```python
from build123d import *

# Parameters (mm, degrees)
SKETCH1_W           = 26.67
SKETCH1_H           = 6.858
BOSS_EXTRUDE1_DEPTH = 5.588
CUT_EXTRUDE1_REACH  = 184.177
SKETCH9_W           = 6.096
SKETCH9_H           = 12.7
CUT_EXTRUDE2_REACH  = 184.177
SKETCH12_R          = 3.175
CUT_EXTRUDE3_REACH  = 184.177
SKETCH13_R          = 4.445


with BuildPart() as part:
    # Sketch1 → Boss-Extrude1 (new body)
    with BuildSketch(Plane(origin=(0, 0, 0), x_dir=(1, 0, 0), z_dir=(0, 1, 0))):
        Polygon((-110.690062624, 12.380140685), (-116.278062624, 12.380140685), (-116.278062624, 0.950140685), (-110.690062624, 0.950140685), (-110.690062624, -46.674859251), (-97.228062624, -46.674859251), (-97.228062624, -52.262859251), (-85.798062624, -52.262859251), (-85.798062624, -46.674859251), (-59.128062624, -46.674859251), (-59.128062624, -52.262859251), (-15.948062624, -52.262859251), (-15.948062624, -46.674859251), (10.721937376, -46.674859251), (10.721937376, -52.262859251), (72.951937376, -52.262859251), (72.951937376, -46.674859251), (99.621937376, -46.674859251), (99.621937376, -52.262859251), (130.101937376, -52.262859251), (130.101937376, -46.67485938), (143.563937376, -46.67485938), (143.563937376, 0.950140682), (149.151937376, 0.950140682), (149.151937376, 12.38014062), (143.563937376, 12.38014062), (143.563937376, 60.00514062), (130.101937376, 60.00514062), (130.101937376, 66.86314062), (143.563937376, 66.86314062), (143.563937376, 104.45514062), (-105.610062624, 104.45514062), (-105.610062624, 66.86314062), (-97.228062624, 66.86314062), (-97.228062624, 60.00514062), (-110.690062624, 60.00514062), align=None)
        with Locations((-72.463062624, 63.43414062)):
            Rectangle(SKETCH1_W, SKETCH1_H, mode=Mode.SUBTRACT)
        with Locations((-2.613062624, 63.43414062)):
            Rectangle(SKETCH1_W, SKETCH1_H, mode=Mode.SUBTRACT)
        with Locations((86.286937376, 63.43414062)):
            Rectangle(SKETCH1_W, SKETCH1_H, mode=Mode.SUBTRACT)
    extrude(amount=BOSS_EXTRUDE1_DEPTH)

    # Sketch9 → Cut-Extrude1 (cut, up to next)
    with BuildSketch(Plane(origin=(0, 5.588, 0), x_dir=(1, 0, 0), z_dir=(0, 1, 0)), mode=Mode.PRIVATE) as cut_extrude1_sk1:
        with Locations((-20.012062624, -23.687859251)):
            Rectangle(SKETCH9_W, SKETCH9_H)
    cut_extrude1_tool1 = extrude(cut_extrude1_sk1.sketch, amount=-CUT_EXTRUDE1_REACH, mode=Mode.PRIVATE) & part.part
    # Sketch9 → Cut-Extrude1 (cut, up to next)
    with BuildSketch(Plane(origin=(0, 5.588, 0), x_dir=(1, 0, 0), z_dir=(0, 1, 0)), mode=Mode.PRIVATE) as cut_extrude1_sk2:
        with Locations((-20.012062624, 42.860140749)):
            Rectangle(SKETCH9_W, SKETCH9_H)
    cut_extrude1_tool2 = extrude(cut_extrude1_sk2.sketch, amount=-CUT_EXTRUDE1_REACH, mode=Mode.PRIVATE) & part.part
    # Sketch9 → Cut-Extrude1 (cut, up to next)
    with BuildSketch(Plane(origin=(0, 5.588, 0), x_dir=(1, 0, 0), z_dir=(0, 1, 0)), mode=Mode.PRIVATE) as cut_extrude1_sk3:
        with Locations((133.657937376, -23.687859251)):
            Rectangle(SKETCH9_W, SKETCH9_H)
    cut_extrude1_tool3 = extrude(cut_extrude1_sk3.sketch, amount=-CUT_EXTRUDE1_REACH, mode=Mode.PRIVATE) & part.part
    # Sketch9 → Cut-Extrude1 (cut, up to next)
    with BuildSketch(Plane(origin=(0, 5.588, 0), x_dir=(1, 0, 0), z_dir=(0, 1, 0)), mode=Mode.PRIVATE) as cut_extrude1_sk4:
        with Locations((133.657937376, 42.860140749)):
            Rectangle(SKETCH9_W, SKETCH9_H)
    cut_extrude1_tool4 = extrude(cut_extrude1_sk4.sketch, amount=-CUT_EXTRUDE1_REACH, mode=Mode.PRIVATE) & part.part
    add(cut_extrude1_tool1.solids().sort_by_distance((-20.012063, 5.588, 23.687859))[0], mode=Mode.SUBTRACT)
    add(cut_extrude1_tool2.solids().sort_by_distance((-20.012063, 5.588, -42.860141))[0], mode=Mode.SUBTRACT)
    add(cut_extrude1_tool3.solids().sort_by_distance((133.657937, 5.588, 23.687859))[0], mode=Mode.SUBTRACT)
    add(cut_extrude1_tool4.solids().sort_by_distance((133.657937, 5.588, -42.860141))[0], mode=Mode.SUBTRACT)

    # Sketch12 → Cut-Extrude2 (cut, up to next)
    with BuildSketch(Plane(origin=(0, 5.588, 0), x_dir=(1, 0, 0), z_dir=(0, 1, 0)), mode=Mode.PRIVATE) as cut_extrude2_sk1:
        with Locations(Location((-101.165062624, 28.25514062, 0), (0, 0, 270))):
            Circle(SKETCH12_R)
    cut_extrude2_tool1 = extrude(cut_extrude2_sk1.sketch, amount=-CUT_EXTRUDE2_REACH, mode=Mode.PRIVATE) & part.part
    add(cut_extrude2_tool1.solids().sort_by_distance((-101.165063, 5.588, -28.255141))[0], mode=Mode.SUBTRACT)

    # Sketch13 → Cut-Extrude3 (cut, up to next)
    with BuildSketch(Plane.XZ, mode=Mode.PRIVATE) as cut_extrude3_sk1:
        with Locations(Location((77.273937376, 20.297859251, 0), (0, 0, 270))):
            Circle(SKETCH13_R)
    cut_extrude3_tool1 = extrude(cut_extrude3_sk1.sketch, amount=-CUT_EXTRUDE3_REACH, mode=Mode.PRIVATE) & part.part
    # Sketch13 → Cut-Extrude3 (cut, up to next)
    with BuildSketch(Plane.XZ, mode=Mode.PRIVATE) as cut_extrude3_sk2:
        with Locations(Location((55.099783131, -40.95514062, 0), (0, 0, 270))):
            Circle(SKETCH13_R)
    cut_extrude3_tool2 = extrude(cut_extrude3_sk2.sketch, amount=-CUT_EXTRUDE3_REACH, mode=Mode.PRIVATE) & part.part
    # Sketch13 → Cut-Extrude3 (cut, up to next)
    with BuildSketch(Plane.XZ, mode=Mode.PRIVATE) as cut_extrude3_sk3:
        with Locations(Location((94.474354319, -40.95514062, 0), (0, 0, 270))):
            Circle(SKETCH13_R)
    cut_extrude3_tool3 = extrude(cut_extrude3_sk3.sketch, amount=-CUT_EXTRUDE3_REACH, mode=Mode.PRIVATE) & part.part
    # Sketch13 → Cut-Extrude3 (cut, up to next)
    with BuildSketch(Plane.XZ, mode=Mode.PRIVATE) as cut_extrude3_sk4:
        with Locations(Location((75.424354319, -15.55514062, 0), (0, 0, 270))):
            Circle(SKETCH13_R)
    cut_extrude3_tool4 = extrude(cut_extrude3_sk4.sketch, amount=-CUT_EXTRUDE3_REACH, mode=Mode.PRIVATE) & part.part
    # Sketch13 → Cut-Extrude3 (cut, up to next)
    with BuildSketch(Plane.XZ, mode=Mode.PRIVATE) as cut_extrude3_sk5:
        with Locations(Location((29.478937376, -48.367787821, 0), (0, 0, 270))):
            Circle(SKETCH13_R)
    cut_extrude3_tool5 = extrude(cut_extrude3_sk5.sketch, amount=-CUT_EXTRUDE3_REACH, mode=Mode.PRIVATE) & part.part
    add(cut_extrude3_tool1.solids().sort_by_distance((77.273937, 0, 20.297859))[0], mode=Mode.SUBTRACT)
    add(cut_extrude3_tool2.solids().sort_by_distance((55.099783, 0, -40.955141))[0], mode=Mode.SUBTRACT)
    add(cut_extrude3_tool3.solids().sort_by_distance((94.474354, 0, -40.955141))[0], mode=Mode.SUBTRACT)
    add(cut_extrude3_tool4.solids().sort_by_distance((75.424354, 0, -15.555141))[0], mode=Mode.SUBTRACT)
    add(cut_extrude3_tool5.solids().sort_by_distance((29.478937, 0, -48.367788))[0], mode=Mode.SUBTRACT)


solid = part.part
```
Verification items for the finished model (mm, model axes). A direction names the side the tool comes from. Coordinates: 2 decimals unless noted, no trailing zeros. Order: outer loops, then holes, each group sorted by start corner. A loop starts at its lowest first (then second) coordinate and runs counter-clockwise, first axis right, second up. Notation, with made-up numbers: (38, 68) -> (71, 68) arc R29 ccw to (71, 93) -> close; hole circle Ø1 at (-32, 29.25). An arc over 180 degrees is marked (long way). Put each result on its own line as item: value. Start each with the question number.
1) Material ranges on L1, parallel to X at y = 2.05, z = 25.5; L2, parallel to Z at x = -85, y = 0.7; L3, parallel to X at y = 5.1, z = -62, recorded low to high.
2) Cross-section at A-A (x = -9). Enter the section's corners in (y, z), plus the area to 3 significant figures.
3) Tool access check on faces 1 (the flat face through (-110.69, 3, 23)), 2 (the flat face through (-3, 3, -66.863)), 3 (the flat face through (130.102, 3, 50)), 4 (the flat face through (-97.228, 3, -63)), 5 (the flat face through (72.952, 3, 50)). Record the directions out of +Z, -Z, +X, -X, +Y, -Y that give a thin tool (end or side, any length) a straight path to the whole face; none if there is none.
4) Cross-section at B-B (z = 27.5). Enter the section's corners in (x, y), plus the area to 3 significant figures.
5) Cross-section at C-C (z = -63.5). Enter the section's corners in (x, y), plus the area to 3 significant figures.
6) Go/stop test with flat-tipped pins: pin 1 (1.7 mm diameter, centred on y = 1.5, z = 48.5, fed in from +X); pin 2 (3 mm diameter, centred on y = 3.5, z = -88, fed in from +X); pin 3 (2 mm diameter, centred on x = 70, z = -46.5, fed in from -Y); pin 4 (3 mm diameter, centred on x = 91, y = 3, fed in from +Z). Record where each tip stops, or that it passes through.
7) Cross-section at D-D (y = 4). State how many separate pieces and enclosed holes the cut face has, plus the area to 3 significant figures.
8) Release check for a two-part mould opening along Z. For faces 6 (the flat face through (-38, 3, 52.263)), 7 (the flat face through (146, 3, -12.38)), 8 (the flat face through (143.564, 3, 23)), 9 (the flat face through (134, 3, 30.038)) record: pulls with the +Z half, pulls with the -Z half, needs draft (parallel to the pull), parting line crosses it, or undercut.
Geometry check:
1. L1: x = -110.69 to -23.06, -16.96 to 130.61, 136.71 to 143.56
1. L2: z = -104.46 to -66.86, -60.01 to 46.67
1. L3: x = -97.23 to -85.8, -59.13 to -15.95, 10.72 to 72.95, 99.62 to 130.1
2. outline: (0, -104.46) -> (5.59, -104.46) -> (5.59, -66.86) -> (0, -66.86) -> close; (0, -60.01) -> (5.59, -60.01) -> (5.59, 46.67) -> (0, 46.67) -> close
2. area: 806 mm^2
3. face 1: +Z, -X, +Y, -Y
3. face 2: +Y, -Y
3. face 3: +Z, +X, +Y, -Y
3. face 4: -X, +Y, -Y
3. face 5: +Z, +Y, -Y
4. outline: (-110.69, 0) -> (-23.06, 0) -> (-23.06, 5.59) -> (-110.69, 5.59) -> close; (-16.96, 0) -> (130.61, 0) -> (130.61, 5.59) -> (-16.96, 5.59) -> close; (136.71, 0) -> (143.56, 0) -> (143.56, 5.59) -> (136.71, 5.59) -> close
4. area: 1,350 mm^2
5. outline: (-97.23, 0) -> (-85.8, 0) -> (-85.8, 5.59) -> (-97.23, 5.59) -> close; (-59.13, 0) -> (-15.95, 0) -> (-15.95, 5.59) -> (-59.13, 5.59) -> close; (10.72, 0) -> (72.95, 0) -> (72.95, 5.59) -> (10.72, 5.59) -> close; (99.62, 0) -> (130.1, 0) -> (130.1, 5.59) -> (99.62, 5.59) -> close
5. area: 823 mm^2
6. pin 1: stops at x = 130.1
6. pin 2: stops at x = 143.56
6. pin 3: stops at y = 0
6. pin 4: stops at z = 46.67
7. separate pieces: 1
7. enclosed holes: 13
7. area: 37,800 mm^2
8. face 6: pulls with the +Z half
8. face 7: pulls with the -Z half
8. face 8: needs draft
8. face 9: undercut
